Source: CAD feature listing. Evaluate the final solid. Frame: model axes, mm. Round coordinates to 2 decimals unless told otherwise and drop trailing zeros. Order: outer loops, then holes, each group sorted by start corner. A loop starts at its lowest first (then second) coordinate and runs counter-clockwise, first axis right, second up. Notation, with made-up numbers: (43.25, 36.25) -> (59.25, 36.25) arc R19 ccw to (59.25, 72.25) -> close; hole circle Ø9 at (89, -12). An arc over 180 degrees is marked (long way). Write item = value, one per line. Start each with the question number.
(1) Cut plane B-B on x = -41.5. Return the cut outline in (y, z).
(2) Cut plane A-A on x = 30. Return the cut outline in (y, z), then the cut area to 3 significant figures.
(3) Ray query, line 1 (X direction, y = 42.5, z = 0.35); line 2 (Y direction, x = -37, z = 0.1); line 3 (Y direction, x = -28, z = 0.35). Return the intervals inside material, ascending.
from build123d import *

# Parameters (mm, degrees)
F1_DEPTH = 0.4


with BuildPart() as f1:
    # F0 (on Top) → F1 (new body)
    with BuildSketch(Plane.XY):
        Polygon((14.694631, 20.225425), (0, 40), (-14.694631, 20.225425), (-38.042261, 12.36068), (-23.776413, -7.725425), (-23.51141, -32.36068), (-23.51141, -36.552122), (0, -29.191442), (27.453279, -37.786197), (27.762712, -9.020652), (44.420338, 14.433043), (17.158299, 23.616373), (0, 46.706308), (-17.158299, 23.616373), (-44.420338, 14.433043), (-27.762712, -9.020652), (-27.453279, -37.786197), (-27.453279, -41.977639), (0, -33.382885), (31.395148, -43.211714), (31.74901, -10.315879), (50.798416, 16.505406), (19.621967, 27.007321), (0, 53.412616), (-19.621967, 27.007321), (-50.798416, 16.505406), (-31.74901, -10.315879), (-31.395148, -43.211714), (-28.438746, -42.286158), (-28.438746, -39.142576), (-28.759286, -9.344459), (-46.014858, 14.951134), (-17.774216, 24.46411), (0, 48.382885), (17.774216, 24.46411), (46.014858, 14.951134), (28.759286, -9.344459), (28.438746, -39.142576), (0, -30.239303), (-24.496877, -37.908501), (-24.496877, -33.717059), (-24.772988, -8.049232), (-39.63678, 12.878771), (-15.310548, 21.073162), (0, 41.676577), (15.310548, 21.073162), (39.63678, 12.878771), (24.772988, -8.049232), (24.496877, -33.717059), (0, -26.047861), (-20.510072, -32.468916), (-20.555008, -28.291542), (-20.786689, -6.754005), (-33.258702, 10.806407), (-12.84688, 17.682214), (0, 34.970269), (12.84688, 17.682214), (33.258702, 10.806407), (20.786689, -6.754005), (20.555008, -28.291542), (0, -21.856418), (-16.568203, -27.043399), (-16.61314, -22.866025), (-16.80039, -5.458778), (-26.880625, 8.734044), (-10.383212, 14.291266), (0, 28.263961), (10.383212, 14.291266), (26.880625, 8.734044), (16.80039, -5.458778), (16.61314, -22.866025), (0, -17.664976), (-12.626335, -21.617882), (-12.671271, -17.440508), (-12.814092, -4.163551), (-20.502547, 6.661681), (-7.919544, 10.900318), (0, 21.557654), (7.919544, 10.900318), (20.502547, 6.661681), (12.814092, -4.163551), (12.671271, -17.440508), (0, -13.473533), (-8.684466, -16.192365), (-8.729402, -12.014991), (-8.827793, -2.868324), (-14.124469, 4.589318), (-5.455876, 7.509369), (0, 14.851346), (5.455876, 7.509369), (14.124469, 4.589318), (8.827793, -2.868324), (8.729402, -12.014991), (0, -9.282091), (-4.742597, -10.766848), (-4.787533, -6.589474), (-4.841495, -1.573097), (-7.746391, 2.516955), (-2.992208, 4.118421), (0, 8.145038), (2.992208, 4.118421), (7.746391, 2.516955), (4.841495, -1.573097), (4.787533, -6.589474), (0, -5.090649), (-0.800728, -5.341331), (-0.811962, -4.296988), (0, -4.042788), (3.802066, -5.233095), (3.84492, -1.24929), (6.151872, 1.998864), (2.376291, 3.270684), (0, 6.468461), (-2.376291, 3.270684), (-6.151872, 1.998864), (-3.84492, -1.24929), (-3.802066, -5.233095), (-3.75713, -9.410469), (0, -8.23423), (7.743935, -10.658612), (7.831219, -2.544517), (12.52995, 4.071227), (4.839959, 6.661632), (0, 13.174769), (-4.839959, 6.661632), (-12.52995, 4.071227), (-7.831219, -2.544517), (-7.743935, -10.658612), (-7.698999, -14.835986), (0, -12.425673), (11.685804, -16.084129), (11.817517, -3.839744), (18.908027, 6.143591), (7.303627, 10.05258), (0, 19.881077), (-7.303627, 10.05258), (-18.908027, 6.143591), (-11.817517, -3.839744), (-11.685804, -16.084129), (-11.640867, -20.261503), (0, -16.617115), (15.627672, -21.509646), (15.803816, -5.134971), (25.286105, 8.215954), (9.767295, 13.443529), (0, 26.587384), (-9.767295, 13.443529), (-25.286105, 8.215954), (-15.803816, -5.134971), (-15.627672, -21.509646), (-15.582736, -25.68702), (0, -20.808558), (19.569541, -26.935163), (19.790114, -6.430198), (31.664183, 10.288317), (12.230963, 16.834477), (0, 33.293692), (-12.230963, 16.834477), (-31.664183, 10.288317), (-19.790114, -6.430198), (-19.569541, -26.935163), (-19.524605, -31.112537), (0, -25), (23.51141, -32.36068), (23.776413, -7.725425), (38.042261, 12.36068), align=None)
    extrude(amount=F1_DEPTH)


solid = f1.part
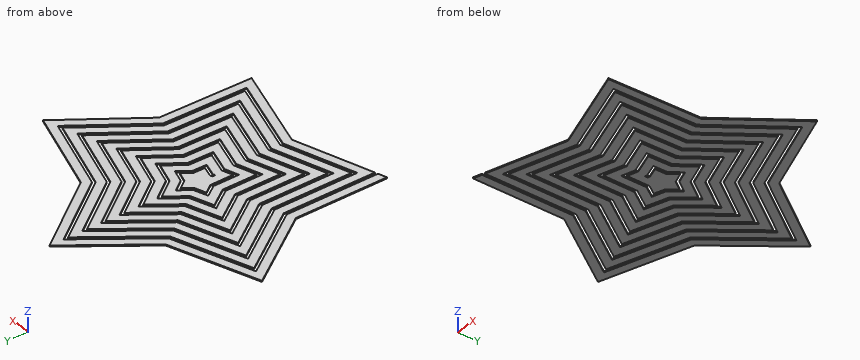
Evaluation:
q1.outline = (3.41, 0) -> (8.59, 0) -> (8.59, 0.4) -> (3.41, 0.4) -> close; (10.32, 0) -> (15.42, 0) -> (15.42, 0.4) -> (10.32, 0.4) -> close; (16.47, 0) -> (19.64, 0) -> (19.64, 0.4) -> (16.47, 0.4) -> close
q2.outline = (-42.77, 0) -> (-7.6, 0) -> (-7.6, 0.4) -> (-42.77, 0.4) -> close; (-5.87, 0) -> (-0.69, 0) -> (-0.69, 0.4) -> (-5.87, 0.4) -> close; (1.04, 0) -> (6.22, 0) -> (6.22, 0.4) -> (1.04, 0.4) -> close; (7.95, 0) -> (10.85, 0) -> (10.85, 0.4) -> (7.95, 0.4) -> close; (11.9, 0) -> (15.07, 0) -> (15.07, 0.4) -> (11.9, 0.4) -> close; (16.12, 0) -> (19.29, 0) -> (19.29, 0.4) -> (16.12, 0.4) -> close; (20.35, 0) -> (23.51, 0) -> (23.51, 0.4) -> (20.35, 0.4) -> close
q2.area = 23.2 mm^2
q3.line_1 = -8.11 to -4.37, -3.13 to 3.13, 4.37 to 8.11
q3.line_2 = -2.92 to 2.26, 3.99 to 9.17, 10.89 to 12.71, 13.77 to 16.93, 17.99 to 21.15
q3.line_3 = -8.69 to -3.51, -1.78 to 3.4, 5.13 to 11.52, 12.58 to 15.74, 16.8 to 19.96, 21.02 to 24.19
